Answer from the drawing. Dimensions are ordinates in mm from the lowest x, y and z of the part. A direction names the side the tool comes from. Round coordinates to 2 decimals unless told otherwise and drop trailing zeros. Loops run counter-clockwise (first coordinate to the right, second up) from the corner with the lowest first, then second, coordinate; pieces in that order, holes last.
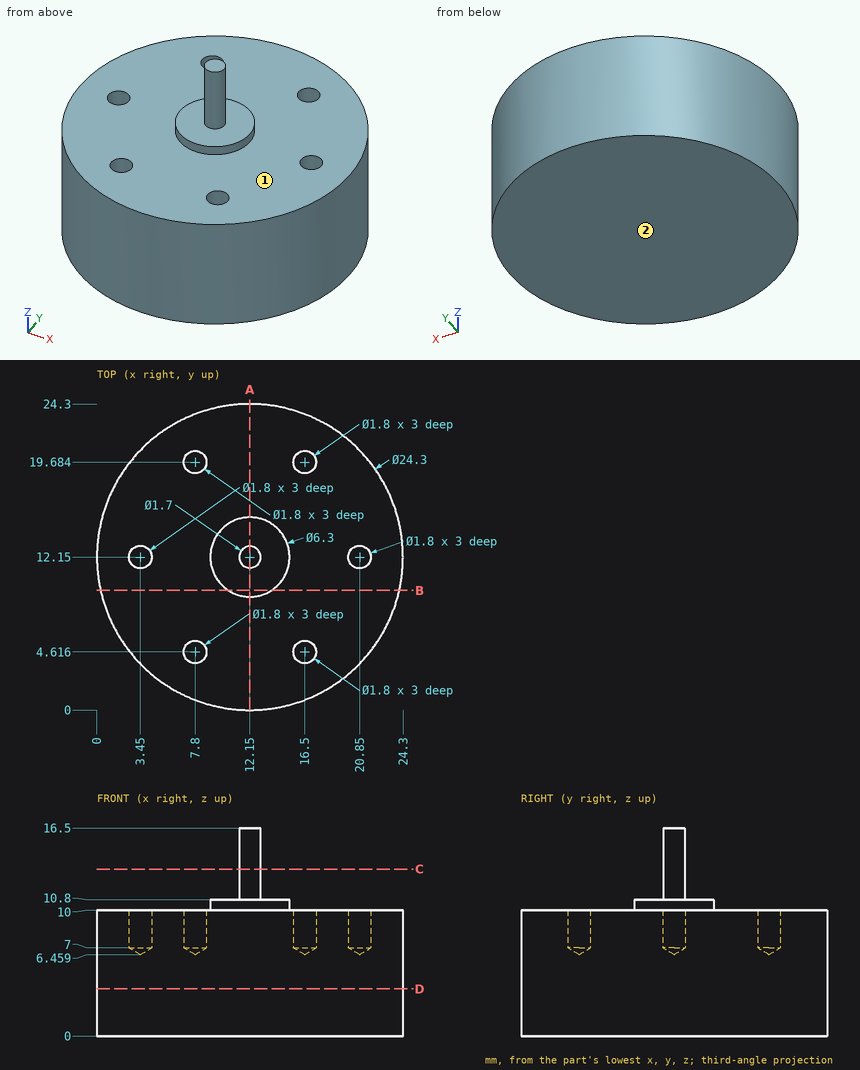
Item 1: For the marked faces 1 and 2, determine the directions among +Z, -Z, +X, -X, +Y, -Y from which every point of the face is accessible in a straight line to the end or side of a thin tool.
Item 2: Section C-C, the plane z = 13.25 is taken. Give the vertices of the cut face in (x, y).
Item 3: Each of these flat-tipped pins is pushed along its axis until it touches: P1, Ø5, axis at x = 17, y = 20.5, coming from the +Z side; P2, Ø1.1, axis at x = 20.85, y = 12.15, coming from the +Z side; P3, Ø5, axis at x = 21.5, z = 7.5, coming from the +Y side (1 decimal); P4, Ø7.5, axis at x = 10, y = 13, coming from the +Z side. Where does it stop, or does it pass through?
Item 4: Straight lines are drawn through the part: line 1 (Y direction, x = 7.8, z = 9.3) (1 decimal); line 2 (Z direction, x = 11.25, y = 19); line 3 (Z direction, x = 14.75, y = 13.5). For each, find the intervals that lie inside material, in ascending order.
Item 5: Section B-B, the plane y = 9.5 is taken. Give the vertices of the cut face in (x, z).
Item 6: Section D-D, the plane z = 3.75 is taken. Give the vertices of the cut face in (x, y), plus the area to 3 significant figures.
Item 7: Section A-A, the plane x = 12.15 is taken. Give the vertices of the cut face in (y, z).
Answer below:
1. face 1: +Z
1. face 2: -Z, +X, -X, +Y, -Y
2. outline: circle Ø1.7 at (12.15, 12.15)
3. P1: stops at z = 10
3. P2: stops at z = 6.79
3. P3: stops at y = 22.2
3. P4: stops at z = 16.5
4. line 1: y = 0.8 to 3.7, 5.5 to 18.8, 20.6 to 23.5
4. line 2: z = 0 to 10
4. line 3: z = 0 to 10.8
5. outline: (0.29, 0) - (24.01, 0) - (24.01, 10) - (13.85, 10) - (13.85, 10.8) - (10.45, 10.8) - (10.45, 10) - (0.29, 10) - close
6. outline: circle Ø24.3 at (12.15, 12.15)
6. area: 464 mm2
7. outline: (0, 0) - (24.3, 0) - (24.3, 10) - (15.3, 10) - (15.3, 10.8) - (13, 10.8) - (13, 16.5) - (11.3, 16.5) - (11.3, 10.8) - (9, 10.8) - (9, 10) - (0, 10) - close
